from build123d import *

# Parameters (mm, degrees)
F0_W      = 51
F0_H      = 14
F1_DEPTH  = 6
F2_R      = 2.5
F3_DEPTH  = 4
F6_DEPTH  = 2
F7_DEPTH  = 3
F8_W      = 10
F8_H      = 9
F9_DEPTH  = 10
F10_W     = 10
F10_H     = 10
F11_DEPTH = 25
F12_W     = 10.0145330653
F12_H     = 9
F12_W_2   = 10.0145321339
F13_DEPTH = 10
F14_W     = 10.0145330653
F14_H     = 10
F14_W_2   = 10.0145321339
F15_DEPTH = 25
F16_W     = 14
F16_H     = 18
F16_R     = 5.5
F17_DEPTH = 40
F18_R     = 1.7
F19_DEPTH = 5
F20_R     = 2.5
F21_DEPTH = 20
F22_SIZE2 = 5
F22_SIZE  = 10


with BuildPart() as f1:
    # F0 (on Top) → F1 (new body)
    with BuildSketch(Plane.XY):
        Rectangle(F0_W, F0_H)
    extrude(amount=F1_DEPTH)

    # F2 (on face) → F3 (cut)
    with BuildSketch(Plane(origin=(0, 0, 0), x_dir=(1, 0, 0), z_dir=(0, 0, -1))):
        with BuildLine():
            ThreePointArc((0.4634146341, 4.7273403597), (-4.38e-08, 4.75), (-0.4634147213, 4.7273403512))
            ThreePointArc((-0.4634147213, 4.7273403512), (-4.75, -4.38e-08), (-0.4634146341, -4.7273403597))
            ThreePointArc((-0.4634146341, -4.7273403597), (0, -4.75), (0.4634146341, -4.7273403597))
            ThreePointArc((0.4634146341, -4.7273403597), (3.5187866881, -3.1907115576), (4.75, 0))
            ThreePointArc((4.75, 0), (3.5187866881, 3.1907115576), (0.4634146341, 4.7273403597))
        make_face()
        Circle(F2_R, mode=Mode.SUBTRACT)
        Circle(F2_R)
    extrude(amount=-F3_DEPTH, mode=Mode.SUBTRACT)

    # F5 (on offset) → F6 (cut)
    with BuildSketch(Plane(origin=(0, 0, 4), x_dir=(1, 0, 0), z_dir=(0, 0, -1))):
        with BuildLine():
            Line((-0.4634146341, 4.7273403597), (-20.7682926829, 2.7368812609))
            ThreePointArc((-20.7682926829, 2.7368812609), (-23.25, 0), (-20.7682926829, -2.7368812609))
            Line((-20.7682926829, -2.7368812609), (-0.4634146341, -4.7273403597))
            ThreePointArc((-0.4634146341, -4.7273403597), (-4.75, 0), (-0.4634146341, 4.7273403597))
        make_face()
        with BuildLine():
            ThreePointArc((0.4634146341, 4.7273403597), (0, 4.75), (-0.4634146341, 4.7273403597))
            ThreePointArc((-0.4634146341, 4.7273403597), (-4.75, 0), (-0.4634146341, -4.7273403597))
            ThreePointArc((-0.4634146341, -4.7273403597), (0, -4.75), (0.4634146341, -4.7273403597))
            ThreePointArc((0.4634146341, -4.7273403597), (3.5187866881, -3.1907115576), (4.75, 0))
            ThreePointArc((4.75, 0), (3.5187866881, 3.1907115576), (0.4634146341, 4.7273403597))
        make_face()
        with BuildLine():
            Line((20.7682926829, 2.7368812609), (0.4634146341, 4.7273403597))
            ThreePointArc((0.4634146341, 4.7273403597), (3.5187866881, 3.1907115576), (4.75, 0))
            ThreePointArc((4.75, 0), (3.5187866881, -3.1907115576), (0.4634146341, -4.7273403597))
            Line((0.4634146341, -4.7273403597), (20.7682926829, -2.7368812609))
            ThreePointArc((20.7682926829, -2.7368812609), (23.25, 0), (20.7682926829, 2.7368812609))
        make_face()
    extrude(amount=-F6_DEPTH, mode=Mode.SUBTRACT)

    # F7 (add): a face of the model
    f7_faces = [f1.faces().sort_by_distance(p)[0] for p in [
        (0, 6.4711332871, 6),
    ]]
    extrude(f7_faces, amount=F7_DEPTH)

    # F8 (on face) → F9 (join)
    with BuildSketch(Plane.XZ.offset(7)):
        with Locations((15, 4.5)):
            Rectangle(F8_W, F8_H)
        with Locations((-15, 4.5)):
            Rectangle(F8_W, F8_H)
        Polygon((0, 0), (5, 0), (5, 9), (-5, 9), (-5, 0), align=None)
    extrude(amount=F9_DEPTH)

    # F10 (on face) → F11 (join)
    with BuildSketch(Plane.XY.offset(9)):
        with Locations((15, -12)):
            Rectangle(F10_W, F10_H)
        with Locations((0, -12)):
            Rectangle(F10_W, F10_H)
        with Locations((-15, -12)):
            Rectangle(F10_W, F10_H)
    extrude(amount=F11_DEPTH)

    # F12 (on face) → F13 (join)
    with BuildSketch(Plane(origin=(0, 7, 0), x_dir=(-1, 0, 0), z_dir=(0, 1, 0))):
        with Locations((-15.0052965619, 4.5)):
            Rectangle(F12_W, F12_H)
        with Locations((0.0165025704, 4.5)):
            Rectangle(F12_W_2, F12_H)
        with Locations((15.0112351403, 4.5)):
            Rectangle(F12_W_2, F12_H)
    extrude(amount=F13_DEPTH)

    # F14 (on face) → F15 (join)
    with BuildSketch(Plane.XY.offset(9)):
        with Locations((15.0052965619, 12)):
            Rectangle(F14_W, F14_H)
        with Locations((-0.0165025704, 12)):
            Rectangle(F14_W_2, F14_H)
        with Locations((-15.0112351403, 12)):
            Rectangle(F14_W_2, F14_H)
    extrude(amount=F15_DEPTH)

    # F16 (on face) → F17 (join)
    with BuildSketch(Plane.YZ.offset(20.0125630945)):
        with Locations((0, 23.4342994317)):
            Rectangle(F16_W, F16_H)
        with Locations((0, 23.444019258)):
            Circle(F16_R, mode=Mode.SUBTRACT)
    extrude(amount=-F17_DEPTH)

    # F18 (on face) → F19 (cut)
    with BuildSketch(Plane.XY.offset(32.4342994317)):
        with Locations((15, 0)):
            Circle(F18_R)
        with Locations((-14.9937184528, 0)):
            Circle(F18_R)
    extrude(amount=-F19_DEPTH, mode=Mode.SUBTRACT)

    # F20 (on face) → F21 (cut)
    with BuildSketch(Plane.XY.offset(32.4342994317)):
        Circle(F20_R)
    extrude(amount=-F21_DEPTH, mode=Mode.SUBTRACT)

    # F22
    f22_edges = [f1.edges().sort_by_distance(p)[0] for p in [
        (15.005297, 17, 0),
        (-0.016503, 17, 0),
        (-15.011235, 17, 0),
        (15, -17, 0),
        (0, -17, 0),
        (-15, -17, 0),
    ]]
    f22_side = f1.faces().sort_by_distance((22.756282, 6.387056, 0))[0]
    chamfer(f22_edges, length=F22_SIZE, length2=F22_SIZE2, reference=f22_side)


solid = f1.part
Read the model definition and answer for the solid it produces. Units are mm, in the model's axes. A direction names the side the tool comes from. Round coordinates to 2 decimals unless told otherwise and drop trailing zeros. Write each loop counter-clockwise with the first axis right and the second up, starting at its lowest first coordinate (ties: lowest second). Pieces come first, ordered by that corner, then holes. Notation, with made-up numbers: (19, 10) - (44, 10) arc R28 cw to (44, 36) - close; hole circle Ø4 at (-0.75, -16.5). An arc over 180 degrees is marked (long way). Use a Markdown table: item, result.
(1) The part is cut by section C-C (x = 15). Write down the section's boundary in (y, z), then the cut area to 3 significant figures.
Reported:
| item | result |
|---|---|
| outline | (-17, 5) - (-7, 0) - (7, 0) - (17, 5) - (17, 34) - (7, 34) - (7, 32.43) - (1.7, 32.43) - (1.7, 28.67) arc R5.5 cw (long way) to (-1.7, 28.67) - (-1.7, 32.43) - (-7, 32.43) - (-7, 34) - (-17, 34) - close; hole (-7, 9) - (-3.3, 9) - (-3.3, 4) - (3.3, 4) - (3.3, 9) - (7, 9) - (7, 14.43) - (-7, 14.43) - close |
| area | 868 mm2 |
(2) The part is cut by section A-A (y = 11). Write down the section's boundary in (x, z), then the cut area to 3 significant figures.
Reported:
| item | result |
|---|---|
| outline | (-20.02, 2) - (-10, 2) - (-10, 34) - (-20.02, 34) - close; (-5.02, 2) - (4.99, 2) - (4.99, 34) - (-5.02, 34) - close; (10, 2) - (20.01, 2) - (20.01, 34) - (10, 34) - close |
| area | 961 mm2 |
(3) The part is cut by section D-D (y = -14). Write down the section's boundary in (x, z).
Reported:
| item | result |
|---|---|
| outline | (-20, 3.5) - (-10, 3.5) - (-10, 34) - (-20, 34) - close; (-5, 3.5) - (5, 3.5) - (5, 34) - (-5, 34) - close; (10, 3.5) - (20, 3.5) - (20, 34) - (10, 34) - close |
(4) Straight lines are drawn through the part: line 1 along X through (y, z) = (-8.5, 13); line 2 along X through (y, z) = (0, 30.1); line 3 along Y through (x, z) = (15, 30). For each, find the intervals that lie inside material, in ascending order. Write a range as [from, to].
Reported:
| item | result |
|---|---|
| line 1 | [-20, -10], [-5, 5], [10, 20] |
| line 2 | [-19.99, -16.69], [-13.29, -2.5], [2.5, 13.3], [16.7, 20.01] |
| line 3 | [-17, -1.7], [1.7, 17] |
(5) Each of these flat-tipped pins is pushed along its axis until it touches: pin 1 Ø2 at (y, z) = (-10, 28.5) entering from +X; pin 2 Ø2 at (y, z) = (-1, 15) entering from -X; pin 3 Ø12 at (x, y) = (-9.5, -2.5) entering from +Z; pin 4 Ø5 at (x, y) = (-13, 12.5) entering from -Z. Where does it stop, or does it pass through?
Reported:
| item | result |
|---|---|
| pin 1 | x = 20 |
| pin 2 | x = -19.99 |
| pin 3 | z = 34 |
| pin 4 | z = 1.5 |
(6) The mould has two halves that part along Z. Classify faces 6 (the flat face through (15, -17, 19)), 7 (the flat face through (-10.474, -3.746, 6.465)), 8 (the flat face through (0, -3, 32.434)): released by +Z, released by -Z, zero draft, split by the parting line, or undercut.
Reported:
| item | result |
|---|---|
| face 6 | zero draft |
| face 7 | undercut |
| face 8 | released by +Z |
(7) Which of the six approach directions +Z, -Z, +X, -X, +Y, -Y give full straight-line access (tool end or side, diameter ignored) to faces 1 (the flat face through (20.013, 7, 21)), 2 (the flat face through (-10, -12, 17)), 3 (the flat face through (12, 0, 4)), 4 (the cylindrical face through (-23.25, -0.06, 6.46)), 5 (the flat face through (15, -7, 12))?
Reported:
| item | result |
|---|---|
| face 1 | +Z, +X, +Y |
| face 2 | +Z, -Z, -Y |
| face 3 | none |
| face 4 | +Z |
| face 5 | +X, -X |
